Geometry check sheet. Reference: the model listing, model coordinates, mm. Face numbers are marked on the shaded views. A direction names the side the tool comes from. Give positions to 0.01 mm unless a question says otherwise; leave off trailing zeros. Write each loop counter-clockwise with the first axis right and the second up, starting at its lowest first coordinate (ties: lowest second). Pieces come first, ordered by that corner, then holes. Notation, with made-up numbers: (-23.75, -28) -> (15.25, -28) arc R14 ccw to (15.25, -23) -> close; hole circle Ø8 at (53, 25.25). An arc over 180 degrees is marked (long way). One line per item, written item: value.
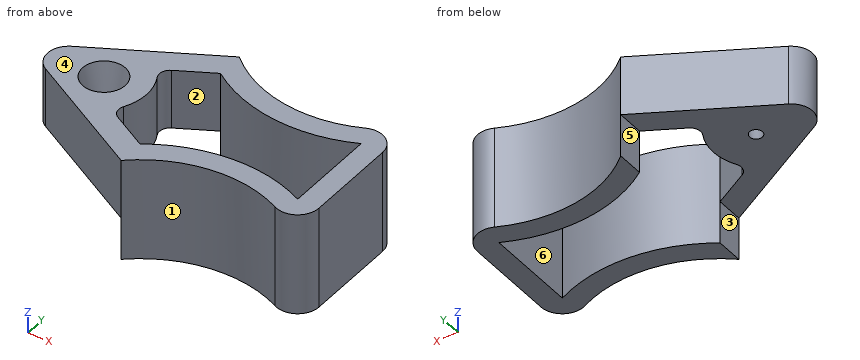
from build123d import *

# Parameters (mm, degrees)
F1_DEPTH = 15.24
F2_R     = 3.175
F5_DEPTH = 15.241
F6_W     = 38.1
F6_H     = 6.35
F7_DEPTH = 25.401


# Not quite as in the source:
# - an extrude whose draft closes it to a point is written as a loft to that point


with BuildPart() as f1:
    # F0 (on Top) → F1 (new body)
    with BuildSketch(Plane.XY):
        with BuildLine():
            ThreePointArc((-25.4, 25.4), (-53.7980633142, 12.7), (-25.4, 0))
            Line((-25.4, 0), (-34.5618496597, 0))
            Line((-34.5618496597, 0), (-34.5618496597, 25.4))
            Line((-34.5618496597, 25.4), (-25.4, 25.4))
        make_face()
        with BuildLine():
            Line((-34.5618496597, 0), (-25.4, 0))
            ThreePointArc((-25.4, 0), (-21.204965459, 5.7439235197), (-19.7203873372, 12.7))
            ThreePointArc((-19.7203873372, 12.7), (-21.204965459, 19.6560764803), (-25.4, 25.4))
            Line((-25.4, 25.4), (-34.5618496597, 25.4))
            Line((-34.5618496597, 25.4), (-34.5618496597, 0))
        make_face()
        with BuildLine():
            ThreePointArc((-19.7203873372, 12.7), (-21.204965459, 5.7439235197), (-25.4, 0))
            ThreePointArc((-25.4, 0), (-15.4225737421, 4.6554132358), (-4.5357142857, 3.0127938932))
            ThreePointArc((-4.5357142857, 3.0127938932), (-1.4778911139, 3.1980667262), (0, 5.8814314849))
            Line((0, 5.8814314849), (0, 19.5185685151))
            ThreePointArc((0, 19.5185685151), (-1.4778911139, 22.2019332738), (-4.5357142857, 22.3872061068))
            ThreePointArc((-4.5357142857, 22.3872061068), (-15.4225737421, 20.7445867642), (-25.4, 25.4))
            ThreePointArc((-25.4, 25.4), (-21.204965459, 19.6560764803), (-19.7203873372, 12.7))
        make_face()
    extrude(amount=F1_DEPTH)

    # F2 (on face) → F3 section 0
    with BuildSketch(Plane.XY.offset(15.24), mode=Mode.PRIVATE) as f3_s0:
        with Locations((-36.7592253257, 12.7)):
            Circle(F2_R)
    loft([f3_s0.sketch, Vertex(-36.7592253257, 12.7, 2.505770536)], ruled=True, mode=Mode.SUBTRACT)

    # F4 (on face) → F5 (cut, through all)
    with BuildSketch(Plane.XY.offset(15.24)):
        with BuildLine():
            ThreePointArc((-25.4, 4.0399547456), (-14.535188109, 7.9500701216), (-3.175, 5.8814314849))
            Line((-3.175, 5.8814314849), (-3.175, 19.5185685151))
            ThreePointArc((-3.175, 19.5185685151), (-14.535188109, 17.4499298784), (-25.4, 21.3600452544))
            Line((-25.4, 21.3600452544), (-30.6912422422, 18.4625566245))
            ThreePointArc((-30.6912422422, 18.4625566245), (-31.4514193427, 17.5192344091), (-31.3248088175, 16.3143710139))
            ThreePointArc((-31.3248088175, 16.3143710139), (-30.4092253257, 12.7), (-31.3248088175, 9.0856289861))
            ThreePointArc((-31.3248088175, 9.0856289861), (-31.4514193427, 7.8807655909), (-30.6912422422, 6.9374433755))
            Line((-30.6912422422, 6.9374433755), (-25.4, 4.0399547456))
        make_face()
        with BuildLine():
            ThreePointArc((-25.4, 25.4), (-53.7980633142, 12.7), (-25.4, 0))
            Line((-25.4, 0), (-43.5066161293, 9.9151979742))
            ThreePointArc((-43.5066161293, 9.9151979742), (-45.1566562358, 12.7), (-43.5066161293, 15.4848020258))
            Line((-43.5066161293, 15.4848020258), (-25.4, 25.4))
        make_face()
    extrude(amount=-F5_DEPTH, mode=Mode.SUBTRACT)

    # F6 (on Front) → F7 (cut, through all)
    with BuildSketch(Plane.XZ):
        with Locations((-44.45, 3.175)):
            Rectangle(F6_W, F6_H)
    extrude(amount=-F7_DEPTH, mode=Mode.SUBTRACT)


solid = f1.part
1) Tool access check on the marked faces 1, 2 and 3. Record the directions out of +Z, -Z, +X, -X, +Y, -Y that give a thin tool (end or side, any length) a straight path to the whole face; none if there is none.
Verdict:
face 1: +Z, -Z, -Y
face 2: +Z, -Z
face 3: -Z, -X, +Y, -Y
2) Sectioned sample at A-A on x = -21. Record the cut outline in (y, z).
Verdict:
outline: (2.95, 0) -> (6.42, 0) -> (6.42, 15.24) -> (2.95, 15.24) -> close; (18.98, 0) -> (22.45, 0) -> (22.45, 15.24) -> (18.98, 15.24) -> close
3) Scan lines: probe 1 along X at (y, z) = (13.25, 7) (1 decimal); probe 2 along X at (y, z) = (14.25, 9.5) (3 decimals); probe 3 along Y at (x, z) = (-9.5, 10). Record each from-to range of solid material in increasing order.
Verdict:
probe 1: -45.1 to -37.7, -35.8 to -30.4, -3.2 to 0
probe 2: -44.753 to -37.558, -35.96 to -30.569, -3.175 to 0
probe 3: 4.58 to 7.79, 17.61 to 20.82
4) Sectioned sample at B-B on z = 7.5. Give the number of separate pieces and of enclosed holes in the cut face, plus the area to 3 significant figures.
Verdict:
separate pieces: 1
enclosed holes: 2
area: 411 mm^2
5) Mould release check, pull along X, two halves, no side actions. Record for the marked faces 4, 5 and 6: released by +X, released by -X, zero draft, split by the parting line, or undercut.
Verdict:
face 4: zero draft
face 5: released by -X
face 6: undercut
6) Sectioned sample at D-D on z = 4.5. Record the cut outline in (x, y) (3 decimals), plus the area to 3 significant figures.
Verdict:
outline: (-25.4, 0) arc R19.05 cw to (-4.536, 3.013) arc R3.175 ccw to (0, 5.881) -> (0, 19.519) arc R3.175 ccw to (-4.536, 22.387) arc R19.05 cw to (-25.4, 25.4) -> (-25.4, 21.36) arc R22.225 ccw to (-3.175, 19.519) -> (-3.175, 5.881) arc R22.225 ccw to (-25.4, 4.04) -> close
area: 209 mm^2
7) Depth check by flat-ended pin: pin 1 Ø10 at (x, y) = (-37.5, 13.5) entering from -Z; pin 2 Ø1 at (x, y) = (-12, 22.5) entering from -Z; pin 3 Ø4 at (x, z) = (-19, 9.5) entering from -Y; pin 4 Ø3 at (y, z) = (23.5, 3.5) entering from -X. Enter the tip coordinate at first touch or a pass-through.
Verdict:
pin 1: z = 6.35
pin 2: through
pin 3: y = 2.95
pin 4: x = -25.4
